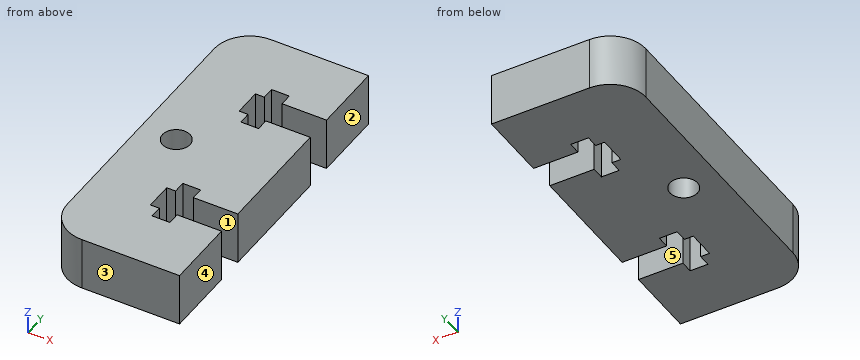
from build123d import *

# Parameters (mm, degrees)
DODANIE_WYCI_GNI_CIE1_DEPTH = 6
WYTNIJ_WYCI_GNI_CIE1_DEPTH  = 15
SZYK_LINIOWY1_COUNT         = 2
SZYK_LINIOWY1_PITCH         = 16.9
SZKIC3_R                    = 1.55
WYTNIJ_WYCI_GNI_CIE2_DEPTH  = 15


with BuildPart() as part:
    # Szkic1 → Dodanie-wyciągnięcie1 (new body)
    with BuildSketch(Plane(origin=(302.151296802, 0, 0), x_dir=(-1, 0, 0), z_dir=(0, 0, -1))):
        with BuildLine():
            Line((-882.390597923, 236.727796113), (-882.390597923, 200.727796113))
            Line((-882.390597923, 200.727796113), (-871.390597923, 200.727796113))
            ThreePointArc((-871.390597923, 200.727796113), (-868.562170798, 201.899368988), (-867.390597923, 204.727796113))
            Line((-867.390597923, 204.727796113), (-867.390597923, 232.727796113))
            ThreePointArc((-867.390597923, 232.727796113), (-868.562170798, 235.556223238), (-871.390597923, 236.727796113))
            Line((-871.390597923, 236.727796113), (-882.390597923, 236.727796113))
        make_face()
    extrude(amount=DODANIE_WYCI_GNI_CIE1_DEPTH)

    # Szkic2 → Wytnij-wyciągnięcie1 (cut)
    with BuildSketch(Plane(origin=(1169.541894725, 0, -6), x_dir=(1, 0, 0), z_dir=(0, 0, 1))):
        Polygon((15, 228.727796113), (15, 225.627796113), (10, 225.627796113), (10, 224.252796113), (8, 224.252796113), (8, 225.627796113), (7, 225.627796113), (7, 228.727796113), (8, 228.727796113), (8, 230.102796113), (10, 230.102796113), (10, 228.727796113), align=None)
    wytnij_wyci_gni_cie1 = extrude(amount=WYTNIJ_WYCI_GNI_CIE1_DEPTH, mode=Mode.SUBTRACT)

    # Szyk liniowy1: Wytnij-wyciągnięcie1 ×2
    with Locations(*[(0, -i * SZYK_LINIOWY1_PITCH, 0) for i in range(1, SZYK_LINIOWY1_COUNT)]):
        add(wytnij_wyci_gni_cie1, mode=Mode.SUBTRACT)

    # Szkic3 → Wytnij-wyciągnięcie2 (cut)
    with BuildSketch(Plane(origin=(0, 0, -6), x_dir=(-1, 0, 0), z_dir=(0, 0, -1))):
        with Locations((-1173.541894725, 218.727796113)):
            Circle(SZKIC3_R)
    extrude(amount=-WYTNIJ_WYCI_GNI_CIE2_DEPTH, mode=Mode.SUBTRACT)


solid = part.part
Part model, mm, in its own coordinate system. Face numbers are marked on the shaded views. A direction names the side the tool comes from. Coordinates: 2 decimals unless noted, no trailing zeros. Write each loop counter-clockwise with the first axis right and the second up, starting at its lowest first coordinate (ties: lowest second). Pieces come first, ordered by that corner, then holes. Notation, with made-up numbers: (13, 18.5) - (36, 18.5) arc R33 ccw to (36, 47.5) - close; hole circle Ø2 at (80.25, 85.25). An arc over 180 degrees is marked (long way). Put each result on its own line as item: value.
1. Band-saw the part on B-B (x = 1181.25). Write the cut outline in (y, z).
Final values:
outline: (200.73, -6) - (208.73, -6) - (208.73, 0) - (200.73, 0) - close; (211.83, -6) - (225.63, -6) - (225.63, 0) - (211.83, 0) - close; (228.73, -6) - (236.73, -6) - (236.73, 0) - (228.73, 0) - close
2. 3-axis set-ups, long thin cutter, end or side, ignore diameter. For the marked faces 1 and 2: which of +Z, -Z, +X, -X, +Y, -Y reach the whole face in a straight line?
Final values:
face 1: +Z, -Z, +X
face 2: +Z, -Z, +X, +Y, -Y
3. Two-plate mould, pull along Y, no slides. Class the marked faces 3, 4 and 5: +Y half, -Y half, draft (parallel to the pull), parting line (faces both ways), or undercut.
Final values:
face 3: -Y half
face 4: draft
face 5: undercut
4. Probe line 1 along Y through (x, z) = (1183, -4.5); line 2 along X through (y, z) = (212, -3.7); line 3 along Y through (x, z) = (1173.5, -0.4). List the from-to ranges inside material, lowest first. Write a range as [from, to].
Final values:
line 1: y = [200.73, 208.73], [211.83, 225.63], [228.73, 236.73]
line 2: x = [1169.54, 1177.54], [1179.54, 1184.54]
line 3: y = [200.73, 217.18], [220.28, 236.73]
5. Band-saw the part on D-D (x = 1172.5). Write the cut outline in (y, z), then the cut area to 3 significant figures.
Final values:
outline: (200.87, -6) - (217.58, -6) - (217.58, 0) - (200.87, 0) - close; (219.88, -6) - (236.59, -6) - (236.59, 0) - (219.88, 0) - close
area: 201 mm²
6. Band-saw the part on A-A (y = 225). Write the cut outline in (x, z), then the cut area to 3 significant figures.
Final values:
outline: (1169.54, -6) - (1177.54, -6) - (1177.54, 0) - (1169.54, 0) - close; (1179.54, -6) - (1184.54, -6) - (1184.54, 0) - (1179.54, 0) - close
area: 78.0 mm²
7. Flat gauge pin, fed straight in: pin 1 Ø0.9 at (y, z) = (227, -2.5) entering from +X. Where does the tip first touch, or does it go through?
Final values:
pin 1: stops at x = 1176.54
